Here's how the part is built. I have some questions about the finished solid (model axes, mm). Face numbers are marked on the shaded views. A direction names the side the tool comes from. Round coordinates to 2 decimals unless told otherwise and drop trailing zeros. Write each loop counter-clockwise with the first axis right and the second up, starting at its lowest first coordinate (ties: lowest second). Pieces come first, ordered by that corner, then holes. Notation, with made-up numbers: (-0.75, -9.5) -> (16.25, -9.5) arc R8 ccw to (16.25, -5.5) -> close; hole circle Ø1 at (5.25, 35.25). An arc over 180 degrees is marked (long way). Answer in a Markdown table with one row per item.
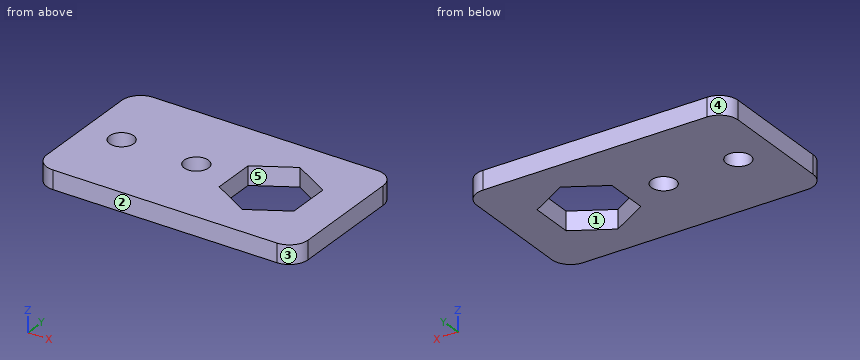
Autodesk Inventor part; units mm, degrees
ref_plane "YZ Plane" through (0, 0, 0) normal (1, 0, 0) x (0, 1, 0)
ref_plane "XZ Plane" through (0, 0, 0) normal (0, 1, 0) x (-1, 0, 0)
ref_plane "XY Plane" through (0, 0, 0) normal (0, 0, 1) x (1, 0, 0)
sketch "Sketch1" plane through (0, 0, 0) normal (0, 0, 1) x (1, 0, 0)
  line L0 (0, 0) -> (44.45, 0)
  line L1 (44.45, 0) -> (44.45, 25.4)
  line L2 (44.45, 25.4) -> (0, 25.4)
  line L3 (0, 25.4) -> (0, 0)
  circle A0 centre (6.35, 12.7) radius 2.0701
  line L4 (31.75, 20.0323) -> (38.1, 16.3662)
  line L5 (38.1, 16.3662) -> (38.1, 9.0338)
  line L6 (38.1, 9.0338) -> (31.75, 5.3677)
  line L7 (31.75, 5.3677) -> (25.4, 9.0338)
  line L8 (25.4, 9.0338) -> (25.4, 16.3662)
  line L9 (25.4, 16.3662) -> (31.75, 20.0323)
  circle A1 centre (19.05, 12.7) radius 2.0701
  point P0 (31.75, 12.7)
  dimension "d0" = 44.45
  dimension "d1" = 25.4
  dimension "d2" = 4.1402
  dimension "d3" = 12.7
  dimension "d4" = 6.35
  dimension "d5" = 25.4
  dimension "d6" = 12.7
  dimension "d7" = 12.7
  dimension "d11" = 12.7
  dimension "d12" = 12.7
extrude "Extrusion1" add sketch "Sketch1" along normal blind 3.175
fillet "Fillet1" radius 3.175 4 edges at (44.45, 25.4, 1.5875) (44.45, 0, 1.5875) (0, 25.4, 1.5875) (0, 0, 1.5875)
properties part number "Hex Spacer 1-2 in (4)" material "Aluminum 6061"
1) I want a section at A-A, the plane y = 12.7. List the corners of the cut face in (x, z) for me (3 decimals).
Response:
| item | result |
|---|---|
| outline | (0, 0) -> (4.28, 0) -> (4.28, 3.175) -> (0, 3.175) -> close; (8.42, 0) -> (16.98, 0) -> (16.98, 3.175) -> (8.42, 3.175) -> close; (21.12, 0) -> (25.4, 0) -> (25.4, 3.175) -> (21.12, 3.175) -> close; (38.1, 0) -> (44.45, 0) -> (44.45, 3.175) -> (38.1, 3.175) -> close |
2) I want a section at D-D, the plane x = 26.5. List the corners of the cut face in (y, z) for me (3 decimals), and give its area (3 significant figures).
Response:
| item | result |
|---|---|
| outline | (0, 0) -> (8.399, 0) -> (8.399, 3.175) -> (0, 3.175) -> close; (17.001, 0) -> (25.4, 0) -> (25.4, 3.175) -> (17.001, 3.175) -> close |
| area | 53.3 mm^2 |
3) We'd pull the mould along X, two halves only. Please class the marked faces 1, 2 and 3: +X half, -X half, draft (parallel to the pull), parting line (faces both ways), or undercut.
Response:
| item | result |
|---|---|
| face 1 | undercut |
| face 2 | draft |
| face 3 | +X half |
4) For pin 1 (3.5 mm diameter, centred on x = 6.35, y = 12.7, fed in from +Z), with a flat end and sliding along its axis, tell me the tip position at first contact or that it passes through.
Response:
| item | result |
|---|---|
| pin 1 | passes through |
5) I need wall thicknesses on line 1 (Y direction, x = 6.35, z = 2.3); line 2 (X direction, y = 15, z = 1.6); line 3 (X direction, y = 19.25, z = 0.75). Which ranges of each line are inside material? Lowest first, please. Write a range as [from, to].
Response:
| item | result |
|---|---|
| line 1 | y = [0, 10.63], [14.77, 25.4] |
| line 2 | x = [0, 25.4], [38.1, 44.45] |
| line 3 | x = [0, 30.39], [33.11, 44.45] |
6) I want a section at C-C, the plane z = 2.1. List the corners of the cut face in (x, y) for me (3 decimals), and give its area (3 significant figures).
Response:
| item | result |
|---|---|
| outline | (0, 3.175) arc R3.175 ccw to (3.175, 0) -> (41.275, 0) arc R3.175 ccw to (44.45, 3.175) -> (44.45, 22.225) arc R3.175 ccw to (41.275, 25.4) -> (3.175, 25.4) arc R3.175 ccw to (0, 22.225) -> close; hole circle Ø4.14 at (6.35, 12.7); hole circle Ø4.14 at (19.05, 12.7); hole (25.4, 9.034) -> (31.75, 5.368) -> (38.1, 9.034) -> (38.1, 16.366) -> (31.75, 20.032) -> (25.4, 16.366) -> close |
| area | 954 mm^2 |
7) I want a section at B-B, the plane x = 19.05. List the corners of the cut face in (y, z) for me (3 decimals), and give its area (3 significant figures).
Response:
| item | result |
|---|---|
| outline | (0, 0) -> (10.63, 0) -> (10.63, 3.175) -> (0, 3.175) -> close; (14.77, 0) -> (25.4, 0) -> (25.4, 3.175) -> (14.77, 3.175) -> close |
| area | 67.5 mm^2 |
8) Which directions (+Z, -Z, +X, -X, +Y, -Y) give clear straight access to the entire face, cutting with the end or side of a thin tool? Please do the marked faces 4 and 5.
Response:
| item | result |
|---|---|
| face 4 | +Z, -Z, -X, +Y |
| face 5 | +Z, -Z |
